```python
from build123d import *

# Parameters (mm, degrees)
SKETCH1_R                                            = 35
SKETCH1_R_2                                          = 8
BOSS_EXTRUDE1_DEPTH                                  = 12
SKETCH2_R                                            = 8
BOSS_EXTRUDE2_DEPTH                                  = 12
BOSS_EXTRUDE3_DEPTH                                  = 12
FILLET1_R                                            = 4
M6_TAPPED_HOLE1_D                                    = 5
CSK_FOR_M6_HEX_SOCKET_COUNTERSUNK_CAP_SC_D           = 6.6
CSK_FOR_M6_HEX_SOCKET_COUNTERSUNK_CAP_SC_CSINK_D     = 13.44
CSK_FOR_M6_HEX_SOCKET_COUNTERSUNK_CAP_SC_CSINK_ANGLE = 90
CSK_FOR_M6_HEX_SOCKET_COUNTERSUNK_CA_2_D             = 6.6
CSK_FOR_M6_HEX_SOCKET_COUNTERSUNK_CA_2_CSINK_D       = 13.44
CSK_FOR_M6_HEX_SOCKET_COUNTERSUNK_CA_2_CSINK_ANGLE   = 90


with BuildPart() as part:
    # Sketch1 → Boss-Extrude1 (new body)
    with BuildSketch(Plane.XY):
        Circle(SKETCH1_R)
        Circle(SKETCH1_R_2, mode=Mode.SUBTRACT)
    extrude(amount=BOSS_EXTRUDE1_DEPTH)

    # Sketch2 → Boss-Extrude2 (add)
    with BuildSketch(Plane.XY.offset(12)):
        with BuildLine():
            Line((15, 25.980762114), (7, 12.124355653))
            ThreePointArc((7, 12.124355653), (14, 0), (7, -12.124355653))
            Line((7, -12.124355653), (15, -25.980762114))
            ThreePointArc((15, -25.980762114), (-30, 0), (15, 25.980762114))
        make_face()
        Circle(SKETCH2_R, mode=Mode.SUBTRACT)
    extrude(amount=BOSS_EXTRUDE2_DEPTH)

    # Sketch5 → Boss-Extrude3 (add)
    with BuildSketch(Plane.XY.offset(12)):
        with BuildLine():
            Line((50, -6), (14, -6))
            ThreePointArc((14, -6), (8, 0), (14, 6))
            Line((14, 6), (50, 6))
            ThreePointArc((50, 6), (56, 0), (50, -6))
        make_face()
    extrude(amount=-BOSS_EXTRUDE3_DEPTH)

    # Fillet1
    fillet1_edges = [part.edges().sort_by_distance(p)[0] for p in [
        (7, -12.124355653, 18),
        (7, 12.124355653, 18),
        (15, 25.980762114, 18),
        (15, -25.980762114, 18),
        (34.481879299, 6, 6),
        (34.481879299, -6, 6),
    ]]
    fillet(fillet1_edges, radius=FILLET1_R)

    # M6 Tapped Hole1 (through all)
    with Locations(Plane.XY.offset(12)):
        with Locations((50, 0)):
            Hole(M6_TAPPED_HOLE1_D / 2)

    # CSK for M6 Hex Socket Countersunk Cap Screw1 (through all)
    with Locations(Plane(origin=(-11, 19.052558883, 24), x_dir=(1, 0, 0), z_dir=(0, 0, 1))):
        with Locations((0, 0), (0, -38.105117766)):
            CounterSinkHole(CSK_FOR_M6_HEX_SOCKET_COUNTERSUNK_CAP_SC_D / 2, CSK_FOR_M6_HEX_SOCKET_COUNTERSUNK_CAP_SC_CSINK_D / 2, counter_sink_angle=CSK_FOR_M6_HEX_SOCKET_COUNTERSUNK_CAP_SC_CSINK_ANGLE)

    # CSK for M6 Hex Socket Countersunk Ca 2 (through all)
    with Locations(Plane(origin=(22, 0, 12), x_dir=(1, 0, 0), z_dir=(0, 0, 1))):
        with Locations((0, 0)):
            CounterSinkHole(CSK_FOR_M6_HEX_SOCKET_COUNTERSUNK_CA_2_D / 2, CSK_FOR_M6_HEX_SOCKET_COUNTERSUNK_CA_2_CSINK_D / 2, counter_sink_angle=CSK_FOR_M6_HEX_SOCKET_COUNTERSUNK_CA_2_CSINK_ANGLE)


solid = part.part
```
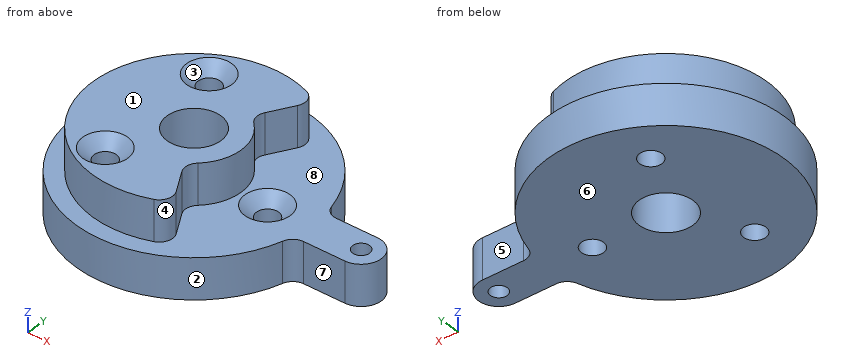
Geometry check sheet. Reference: the model listing, model coordinates, mm. Face numbers are marked on the shaded views. A direction names the side the tool comes from. Coordinates: 2 decimals unless noted, no trailing zeros. Loops run counter-clockwise (first coordinate to the right, second up) from the corner with the lowest first, then second, coordinate; pieces in that order, holes last. Notation, with made-up numbers: (-9.5, 76.5) -> (34.5, 76.5) arc R13 cw to (34.5, 96.5) -> close; hole circle Ø1 at (-24, 29). An arc over 180 degrees is marked (long way). Put each result on its own line as item: value.
1) Gauge pin test, flat ends, axial feed: pin 1 Ø10.5 at (x, y) = (-11, -19.05) entering from -Z; pin 2 Ø6 at (x, z) = (41, 5) entering from -Y; pin 3 Ø12 at (x, z) = (28.5, 6.5) entering from +Y; pin 4 Ø12 at (y, z) = (25.5, 7) entering from +X. Record the tip position at first contact, or that the pin passes through.
Result set:
pin 1: stops at z = 0
pin 2: stops at y = -6
pin 3: stops at y = 26.81
pin 4: stops at x = 29.06
2) Cross-section at B-B on x = 0. Record the boundary of the cut face in (y, z), plus the area to 3 significant figures.
Result set:
outline: (-35, 0) -> (-8, 0) -> (-8, 24) -> (-30, 24) -> (-30, 12) -> (-35, 12) -> close; (8, 0) -> (35, 0) -> (35, 12) -> (30, 12) -> (30, 24) -> (8, 24) -> close
area: 1,180 mm^2
3) Cross-section at C-C on z = 4.25. Record the boundary of the cut face in (x, y), plus the area to 3 significant figures.
Result set:
outline: (33.83, -8.97) arc R4 cw to (37.7, -6) -> (50, -6) arc R6 ccw to (50, 6) -> (37.7, 6) arc R4 cw to (33.83, 8.97) arc R35 ccw (long way) to start; hole circle Ø6.6 at (-11, -19.05); hole circle Ø6.6 at (-11, 19.05); hole circle Ø16 at (0, 0); hole circle Ø6.6 at (22, 0); hole circle Ø5 at (50, 0)
area: 3,770 mm^2
4) Tool access check on the marked faces 4, 5, 6, 7 and 8. Record the directions out of +Z, -Z, +X, -X, +Y, -Y that give a thin tool (end or side, any length) a straight path to the whole face; none if there is none.
Result set:
face 4: +Z, +X
face 5: +Z, -Z, +X, +Y
face 6: -Z, +X, -X, +Y, -Y
face 7: +Z, -Z, +X, -Y
face 8: +Z
5) Thickness scan on line 1 (Y direction, x = -11, z = 12.25); line 2 (Y direction, x = -13, z = 8); line 3 (Y direction, x = 0.5, z = 9.5). Record the ranges inside material, lowest first.
Result set:
line 1: y = -27.91 to -22.35, -15.75 to 15.75, 22.35 to 27.91
line 2: y = -32.5 to -21.68, -16.43 to 16.43, 21.68 to 32.5
line 3: y = -35 to -7.98, 7.98 to 35
6) Cross-section at D-D on z = 15.5. Record the boundary of the cut face in (x, y), plus the area to 3 significant figures.
Result set:
outline: (8.77, -15.2) arc R4 cw to (9.52, -10.27) arc R14 ccw to (9.52, 10.27) arc R4 cw to (8.77, 15.2) -> (12.85, 22.25) arc R4 ccw to (10.82, 27.98) arc R30 ccw (long way) to (10.82, -27.98) arc R4 ccw to (12.85, -22.25) -> close; hole circle Ø6.6 at (-11, -19.05); hole circle Ø6.6 at (-11, 19.05); hole circle Ø16 at (0, 0)
area: 1,820 mm^2
7) Release check for a two-part mould opening along Y. For the marked faces 1, 2 and 3 record: released by +Y, released by -Y, zero draft, split by the parting line, or undercut.
Result set:
face 1: zero draft
face 2: split by the parting line
face 3: undercut
8) Cross-section at A-A on y = 0. Record the boundary of the cut face in (x, z), plus the area to 3 significant figures.
Result set:
outline: (-35, 0) -> (-8, 0) -> (-8, 24) -> (-30, 24) -> (-30, 12) -> (-35, 12) -> close; (8, 0) -> (18.7, 0) -> (18.7, 8.58) -> (15.28, 12) -> (14, 12) -> (14, 24) -> (8, 24) -> close; (25.3, 0) -> (47.5, 0) -> (47.5, 12) -> (28.72, 12) -> (25.3, 8.58) -> close; (52.5, 0) -> (56, 0) -> (56, 12) -> (52.5, 12) -> close
area: 1,090 mm^2
